Geometry check sheet. Reference: the model listing, model coordinates, mm. A direction names the side the tool comes from. Give positions to 0.01 mm unless a question says otherwise; leave off trailing zeros. Write each loop counter-clockwise with the first axis right and the second up, starting at its lowest first coordinate (ties: lowest second). Pieces come first, ordered by that corner, then holes. Notation, with made-up numbers: (-11.5, -14.5) -> (41.5, -14.5) arc R17 ccw to (41.5, 1.5) -> close; hole circle Ø1 at (10, 19). An arc over 180 degrees is marked (long way). One line per item, written item: value.
from build123d import *

# Parameters (mm, degrees)
SKETCH1_W           = 42
SKETCH1_H           = 42
BOSS_EXTRUDE1_DEPTH = 24.5
CHAMFER1_SIZE       = 4
SKETCH2_R           = 11
BOSS_EXTRUDE2_DEPTH = 2
CUT_EXTRUDE1_START  = -0.5
SKETCH3_R           = 16
SKETCH3_R_2         = 11
CUT_EXTRUDE1_DEPTH  = 0.5
SKETCH4_R           = 2.5
BOSS_EXTRUDE3_DEPTH = 22
SKETCH5_W           = 10.364275964
SKETCH5_H           = 1.526028363
CUT_EXTRUDE2_DEPTH  = 20
CIRPATTERN1_COUNT   = 4
FILLET1_R           = 3
CHAMFER2_SIZE       = 0.5
FILLET2_R           = 1
FILLET3_R           = 0.5
SKETCH8_R           = 0.65
BOSS_EXTRUDE4_DEPTH = 2
SKETCH9_R           = 3.5
CUT_EXTRUDE3_DEPTH  = 3.5
BOSS_EXTRUDE5_START = 18.5
SKETCH10_R          = 2.5
BOSS_EXTRUDE5_DEPTH = 18.5
CUT_EXTRUDE4_DEPTH  = 14
CHAMFER3_SIZE       = 0.5


with BuildPart() as part:
    # Sketch1 → Boss-Extrude1 (new, symmetric)
    with BuildSketch(Plane.XY):
        Rectangle(SKETCH1_W, SKETCH1_H)
    extrude(amount=BOSS_EXTRUDE1_DEPTH, both=True)

    # Chamfer1
    chamfer1_edges = [part.edges().sort_by_distance(p)[0] for p in [
        (21, -21, 0),
        (-21, -21, 0),
        (-21, 21, 0),
        (21, 21, 0),
    ]]
    chamfer(chamfer1_edges, length=CHAMFER1_SIZE)

    # Sketch2 → Boss-Extrude2 (add)
    with BuildSketch(Plane.XY.offset(24.5)):
        with Locations(Location((0, 0, 0), (0, 0, 180))):
            Circle(SKETCH2_R)
    extrude(amount=BOSS_EXTRUDE2_DEPTH)

    # Sketch3 → Cut-Extrude1 (cut)
    with BuildSketch(Plane.XY.offset(24.5).offset(CUT_EXTRUDE1_START)):
        Circle(SKETCH3_R)
        Circle(SKETCH3_R_2, mode=Mode.SUBTRACT)
    extrude(amount=CUT_EXTRUDE1_DEPTH, mode=Mode.SUBTRACT)

    # Sketch4 → Boss-Extrude3 (add)
    with BuildSketch(Plane.XY.offset(26.5)):
        Circle(SKETCH4_R)
    extrude(amount=BOSS_EXTRUDE3_DEPTH)

    # Sketch5 → Cut-Extrude2 (cut)
    with BuildSketch(Plane.XY.offset(48.5)):
        with Locations((0.738499094, 2.763014181)):
            Rectangle(SKETCH5_W, SKETCH5_H)
    extrude(amount=-CUT_EXTRUDE2_DEPTH, mode=Mode.SUBTRACT)

    # Sketch7 → M3x0.5 Tapped Hole1 (revolve, cut)
    with BuildSketch(Plane(origin=(-15.5, 15.5, 24.5), x_dir=(0, -1, 0), z_dir=(1, 0, 0))):
        Polygon((0, 0), (0, 8.251075774), (1.25, 7.5), (1.25, 0), align=None)
    m3x0_5_tapped_hole1 = revolve(axis=Axis((-15.5, 15.5, 30.85), (0, 0, -1)), mode=Mode.SUBTRACT)

    # CirPattern1: M3x0.5 Tapped Hole1 ×4 about axis
    cirpattern1_axis = Axis((0, 0, 0), (0, 0, 1))
    for i in range(1, CIRPATTERN1_COUNT):
        add(m3x0_5_tapped_hole1.rotate(cirpattern1_axis, i * 360 / CIRPATTERN1_COUNT), mode=Mode.SUBTRACT)

    # Fillet1
    fillet1_edges = [part.edges().sort_by_distance(p)[0] for p in [
        (17, -21, 0),
        (-17, -21, 0),
        (-21, 17, 0),
        (-21, -17, 0),
        (21, 17, 0),
        (21, -17, 0),
        (17, 21, 0),
        (-17, 21, 0),
    ]]
    fillet(fillet1_edges, radius=FILLET1_R)

    # Chamfer2
    chamfer2_edges = [part.edges().sort_by_distance(p)[0] for p in [
        (-1.118033989, -2.236067977, 48.5),
        (11, 0, 26.5),
    ]]
    chamfer(chamfer2_edges, length=CHAMFER2_SIZE - 0.0001)  # a hair under: the kernel refuses the full size

    # Fillet2
    fillet2_edges = [part.edges().sort_by_distance(p)[0] for p in [
        (-19, -19, -24.5),
        (0, -21, -24.5),
        (-19, 19, -24.5),
        (0, 21, -24.5),
        (19, 19, -24.5),
        (21, 0, -24.5),
        (19, -19, -24.5),
        (-16.90540961, 20.771638598, -24.5),
        (-20.771638598, 16.90540961, -24.5),
        (16.90540961, 20.771638598, -24.5),
        (20.771638598, 16.90540961, -24.5),
        (20.771638598, -16.90540961, -24.5),
        (16.90540961, -20.771638598, -24.5),
        (-16.90540961, -20.771638598, -24.5),
        (-20.771638598, -16.90540961, -24.5),
        (-21, 0, -24.5),
    ]]
    fillet(fillet2_edges, radius=FILLET2_R)

    # Fillet3
    fillet3_edges = [part.edges().sort_by_distance(p)[0] for p in [
        (-16.90540961, 20.771638598, 24.5),
        (-20.771638598, 16.90540961, 24.5),
        (16.90540961, 20.771638598, 24.5),
        (20.771638598, 16.90540961, 24.5),
        (20.771638598, -16.90540961, 24.5),
        (16.90540961, -20.771638598, 24.5),
        (-16.90540961, -20.771638598, 24.5),
        (-20.771638598, -16.90540961, 24.5),
        (-21, 0, 24.5),
        (-19, -19, 24.5),
        (0, -21, 24.5),
        (19, -19, 24.5),
        (21, 0, 24.5),
        (19, 19, 24.5),
        (0, 21, 24.5),
        (-19, 19, 24.5),
    ]]
    fillet(fillet3_edges, radius=FILLET3_R)

    # Sketch8 → Boss-Extrude4 (add)
    with BuildSketch(Plane.XZ.offset(21)):
        with Locations(Location((0, -18.574359193, 0), (0, 0, 90))):
            Circle(SKETCH8_R)
        with Locations(Location((1.158492333, -19.5, 0), (0, 0, 90))):
            Circle(SKETCH8_R)
        with Locations(Location((0.032430158, -20.352099903, 0), (0, 0, 90))):
            Circle(SKETCH8_R)
        with Locations(Location((-1.136757802, -19.5, 0), (0, 0, 90))):
            Circle(SKETCH8_R)
    extrude(amount=BOSS_EXTRUDE4_DEPTH)

    # Sketch9 → Cut-Extrude3 (cut)
    with BuildSketch(Plane(origin=(0, 0, -24.5), x_dir=(-1, 0, 0), z_dir=(0, 0, -1))):
        Circle(SKETCH9_R)
    extrude(amount=-CUT_EXTRUDE3_DEPTH, mode=Mode.SUBTRACT)

    # Sketch10 → Boss-Extrude5 (add)
    with BuildSketch(Plane(origin=(0, 0, -21), x_dir=(-1, 0, 0), z_dir=(0, 0, -1)).offset(BOSS_EXTRUDE5_START)):
        with Locations(Location((0, 0, 0), (0, 0, 53.130102354))):
            Circle(SKETCH10_R)
    extrude(amount=-BOSS_EXTRUDE5_DEPTH)

    # Sketch11 → Cut-Extrude4 (cut)
    with BuildSketch(Plane(origin=(0, 0, -39.5), x_dir=(-1, 0, 0), z_dir=(0, 0, -1))):
        Polygon((-2.474861219, 1.965641899), (2.844080947, 2.039902832), (0.230053947, 6.606484891), align=None)
    extrude(amount=-CUT_EXTRUDE4_DEPTH, mode=Mode.SUBTRACT)

    # Chamfer3
    chamfer3_edges = [part.edges().sort_by_distance(p)[0] for p in [
        (-0.017450722, -2.499939094, -39.5),
    ]]
    chamfer(chamfer3_edges, length=CHAMFER3_SIZE - 0.0001)  # a hair under: the kernel refuses the full size


solid = part.part
1) Tool access check on faces 4 (the flat face through (0, 2, 39)), 5 (the cylindrical face through (0, -2.5, -30.1)), 6 (the cylindrical face through (-16.345, 16.421, 20.803)). Record the directions out of +Z, -Z, +X, -X, +Y, -Y that give a thin tool (end or side, any length) a straight path to the whole face; none if there is none.
Verdict:
face 4: +Z, +X, -X, +Y
face 5: -Z
face 6: +Z
2) Sectioned sample at B-B on z = -16. Record the cut outline in (x, y).
Verdict:
outline: (-21, -15.76) arc R3 ccw to (-20.12, -17.88) -> (-17.88, -20.12) arc R3 ccw to (-15.76, -21) -> (15.76, -21) arc R3 ccw to (17.88, -20.12) -> (20.12, -17.88) arc R3 ccw to (21, -15.76) -> (21, 15.76) arc R3 ccw to (20.12, 17.88) -> (17.88, 20.12) arc R3 ccw to (15.76, 21) -> (-15.76, 21) arc R3 ccw to (-17.88, 20.12) -> (-20.12, 17.88) arc R3 ccw to (-21, 15.76) -> close
3) Scan lines: probe 1 along Y at (x, z) = (0, -22.85); probe 2 along Y at (x, z) = (-15.5, 21.75); probe 3 along X at (y, z) = (-15, 20). Record each from-to range of solid material in increasing order.
Verdict:
probe 1: -21 to -3.5, -2.5 to 2.5, 3.5 to 21
probe 2: -21 to -16.75, -14.25 to 14.25, 16.75 to 21
probe 3: -21 to -16.65, -14.35 to 14.35, 16.65 to 21
4) Depth check by flat-ended pin: pin 1 Ø2 at (x, y) = (-15.5, -15.5) entering from +Z; pin 2 Ø3.5 at (x, z) = (-0.5, 42) entering from +Y; pin 3 Ø10 at (x, y) = (-3.5, -18) entering from -Z. Enter the tip coordinate at first touch or a pass-through.
Verdict:
pin 1: z = 16.85
pin 2: y = 2
pin 3: z = -24.5
5) Sectioned sample at A-A on x = 12. Record the cut outline in (y, z), plus the area to 3 significant figures.
Verdict:
outline: (-21, -23.5) arc R1 ccw to (-20, -24.5) -> (20, -24.5) arc R1 ccw to (21, -23.5) -> (21, 24) arc R0.5 ccw to (20.5, 24.5) -> (10.58, 24.5) -> (10.58, 24) -> (-10.58, 24) -> (-10.58, 24.5) -> (-20.5, 24.5) arc R0.5 ccw to (-21, 24) -> close
area: 2,050 mm^2
6) Sectioned sample at C-C on z = -27. Record the cut outline in (x, y).
Verdict:
outline: (-1.47, 2.02) arc R2.5 ccw (long way) to (1.53, 1.98) -> close
7) Mould release check, pull along X, two halves, no side actions. Record for faces 1 (the flat face through (0, 0, 48.5)), 2 (the flat face through (-2, -2, -21)), 3 (the conical face through (0.064, -2.135, -39.365)): released by +X, released by -X, zero draft, split by the parting line, or undercut.
Verdict:
face 1: zero draft
face 2: undercut
face 3: split by the parting line
